Can you work these out from the drawing? Everything is in mm from the part's minimum corner. A direction names the side the tool comes from. Give positions to 0.01 mm unless a question says otherwise; leave off trailing zeros. Loops run counter-clockwise (first coordinate to the right, second up) from the corner with the lowest first, then second, coordinate; pieces in that order, holes last. Notation, with made-up numbers: (33.25, -11) -> (67.25, -11) arc R23 cw to (67.25, 1) -> close; hole circle Ø5 at (55, -16). An arc over 180 degrees is marked (long way). Write item = value, one per line. Start each with the question number.
1) I want a section at D-D (x = 12.7). List the corners of the cut face in (y, z) for me.
2) I'm going to push a flat-ended pin straight in: pin 1 Ø3.5 at (x, z) = (12.7, 98) entering from +Y. Where does the tip first touch, or does it pass through?
3) I want a section at A-A (z = 98). List the corners of the cut face in (x, y) for me, and give its area (3 significant figures).
4) On a 3-axis mill with a long thin cutter (end or side, diameter ignored), from which of +Z, -Z, +X, -X, +Y, -Y can I reach the whole of each face in a straight line? I mean the marked faces 5 and 6. Say none if no direction works.
5) I need wall thicknesses on probe 1 along Z at (x, y) = (12.7, 24.7); probe 2 along Y at (x, z) = (17, 89.5). Which ranges of each line are inside material? Lowest first, please. Write a range as from..to.
6) If we mould it in two halves opening along Y, with no side actions, what happens to the marked faces 1, 2, 3 and 4? For each: +Y half, -Y half, draft (parallel to the pull), parting line (faces both ways), or undercut.
7) I want a section at B-B (x = 22). List the corners of the cut face in (y, z) for me, and give its area (3 significant figures).
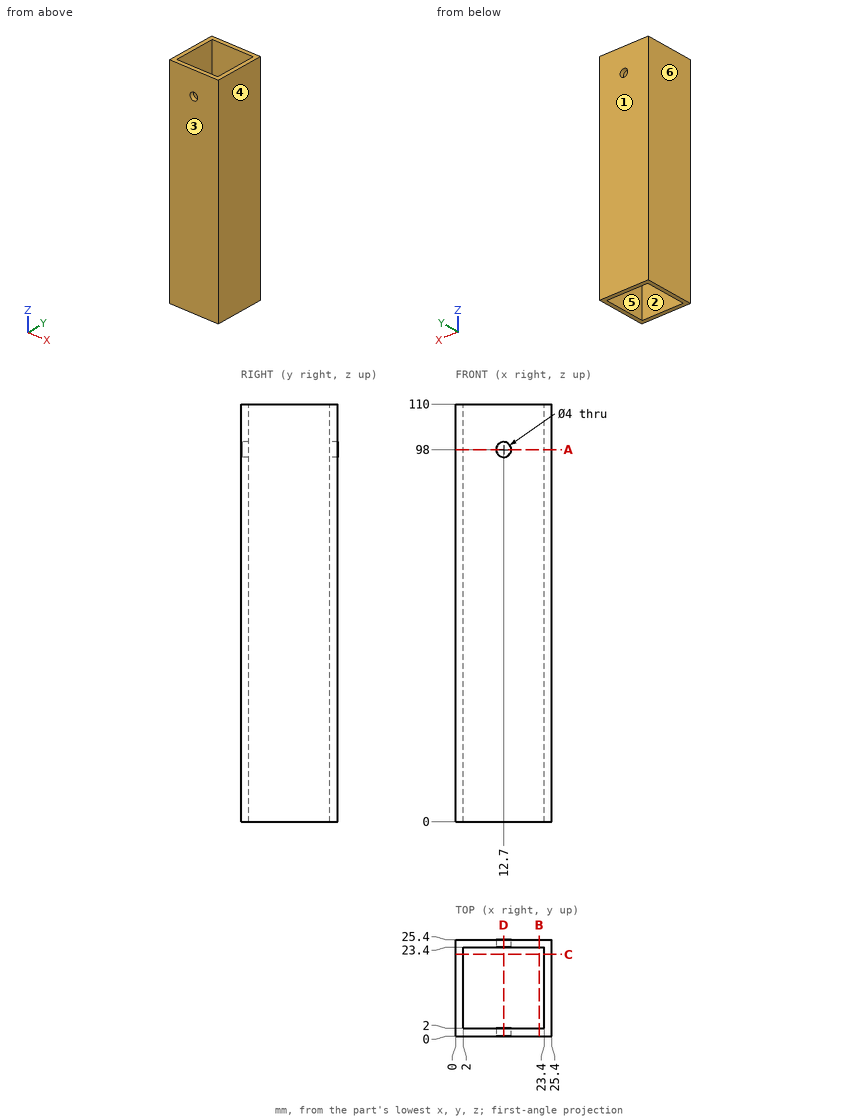
Answer list:
q1.outline = (0, 0) -> (2, 0) -> (2, 96) -> (0, 96) -> close; (0, 100) -> (2, 100) -> (2, 110) -> (0, 110) -> close; (23.4, 0) -> (25.4, 0) -> (25.4, 96) -> (23.4, 96) -> close; (23.4, 100) -> (25.4, 100) -> (25.4, 110) -> (23.4, 110) -> close
q2.pin_1 = through
q3.outline = (0, 0) -> (10.7, 0) -> (10.7, 2) -> (2, 2) -> (2, 23.4) -> (10.7, 23.4) -> (10.7, 25.4) -> (0, 25.4) -> close; (14.7, 0) -> (25.4, 0) -> (25.4, 25.4) -> (14.7, 25.4) -> (14.7, 23.4) -> (23.4, 23.4) -> (23.4, 2) -> (14.7, 2) -> close
q3.area = 171 mm^2
q4.face_5 = +Z, -Z
q4.face_6 = +Z, -Z, -X, +Y, -Y
q5.probe_1 = 0..96, 100..110
q5.probe_2 = 0..2, 23.4..25.4
q6.face_1 = +Y half
q6.face_2 = undercut
q6.face_3 = -Y half
q6.face_4 = draft
q7.outline = (0, 0) -> (2, 0) -> (2, 110) -> (0, 110) -> close; (23.4, 0) -> (25.4, 0) -> (25.4, 110) -> (23.4, 110) -> close
q7.area = 440 mm^2
